Verification items for the finished model (mm, model axes). Round coordinates to 2 decimals unless told otherwise and drop trailing zeros. Order: outer loops, then holes, each group sorted by start corner. A loop starts at its lowest first (then second) coordinate and runs counter-clockwise, first axis right, second up. Notation, with made-up numbers: (-10.75, -16.75) -> (44.25, -16.75) arc R20 ccw to (44.25, 10.25) -> close; hole circle Ø3 at (77, 40). An arc over 180 degrees is marked (long way). Write item = value, one per line. Start each with the question number.
from build123d import *

# Parameters (mm, degrees)
BOSS_EXTRUDE1_DEPTH    = 3.175
SKETCH2_R              = 17.4625
CUT_EXTRUDE1_DEPTH     = 385.384860036
F_10_CLEARANCE_HOLE1_D = 5.1054


with BuildPart() as part:
    # Sketch1 → Boss-Extrude1 (new body)
    with BuildSketch(Plane.XY):
        with BuildLine():
            Line((0, 0), (355.6, 0))
            ThreePointArc((355.6, 0), (381, 25.4), (355.6, 50.8))
            Line((355.6, 50.8), (0, 50.8))
            ThreePointArc((0, 50.8), (-25.4, 25.4), (0, 0))
        make_face()
    extrude(amount=BOSS_EXTRUDE1_DEPTH)

    # Sketch2 → Cut-Extrude1 (cut, through all)
    with BuildSketch(Plane.XY.offset(3.175)):
        with Locations((0, 25.4)):
            Circle(SKETCH2_R)
        with Locations((355.6, 25.4)):
            Circle(SKETCH2_R)
    extrude(amount=-CUT_EXTRUDE1_DEPTH, mode=Mode.SUBTRACT)

    # #10 Clearance Hole1 (through all)
    with Locations(Plane(origin=(18.257547563, 35.941, 3.175), x_dir=(1, 0, 0), z_dir=(0, 0, 1))):
        with Locations((0, 0), (0, -21.082), (-18.257547563, -31.623), (-36.515095126, -21.082), (-36.515095126, 0), (-18.257547563, 10.541)):
            Hole(F_10_CLEARANCE_HOLE1_D / 2)


solid = part.part
(1) Cross-section at C-C (z = 1.05). Give the number of separate pieces and of enclosed holes in the cut face, and give its area (3 significant figures).
(2) Cross-section at A-A (y = 25.4). Enter the section's corners in (x, z) (1 decimal), and give its area (3 significant figures).
(3) Cross-section at B-B (x = 351.5). Enter the section's corners in (y, z) (3 decimals), and give its area (3 significant figures).
(4) Scan lines: line 1 along Y through (x, z) = (0, 0.7); line 2 along X through (y, z) = (25, 2.85); line 3 along X through (y, z) = (27, 2.5). Record each from-to range of solid material in increasing order. Write a range as from..to.
(5) Draft check along X on faces 1 (the cylindrical face through (380.994, 24.841, 1.565)), 2 (the flat face through (175, 26, 0)), 3 (the cylindrical face through (338.154, 26.168, 1.61)). Enter one of: +X half, -X half, draft (parallel to the pull), parting line (faces both ways), or undercut.
(6) Depth check by flat-ended pin: pin 1 (8 mm diameter, centred on x = -18.26, y = 35.94, fed in from +Z) (3 decimals). Enter the tip coordinate at first touch or a pass-through.
Outcome:
q1.separate_pieces = 1
q1.enclosed_holes = 8
q1.area = 18,100 mm^2
q2.outline = (-25.4, 0) -> (-17.5, 0) -> (-17.5, 3.2) -> (-25.4, 3.2) -> close; (17.5, 0) -> (338.1, 0) -> (338.1, 3.2) -> (17.5, 3.2) -> close; (373.1, 0) -> (381, 0) -> (381, 3.2) -> (373.1, 3.2) -> close
q2.area = 1,070 mm^2
q3.outline = (0, 0) -> (8.426, 0) -> (8.426, 3.175) -> (0, 3.175) -> close; (42.374, 0) -> (50.8, 0) -> (50.8, 3.175) -> (42.374, 3.175) -> close
q3.area = 53.5 mm^2
q4.line_1 = 0..1.77, 6.87..7.94, 42.86..43.93, 49.03..50.8
q4.line_2 = -25.4..-17.46, 17.46..338.14, 373.06..381
q4.line_3 = -25.35..-17.39, 17.39..338.21, 372.99..380.95
q5.face_1 = +X half
q5.face_2 = draft
q5.face_3 = undercut
q6.pin_1 = 3.175
